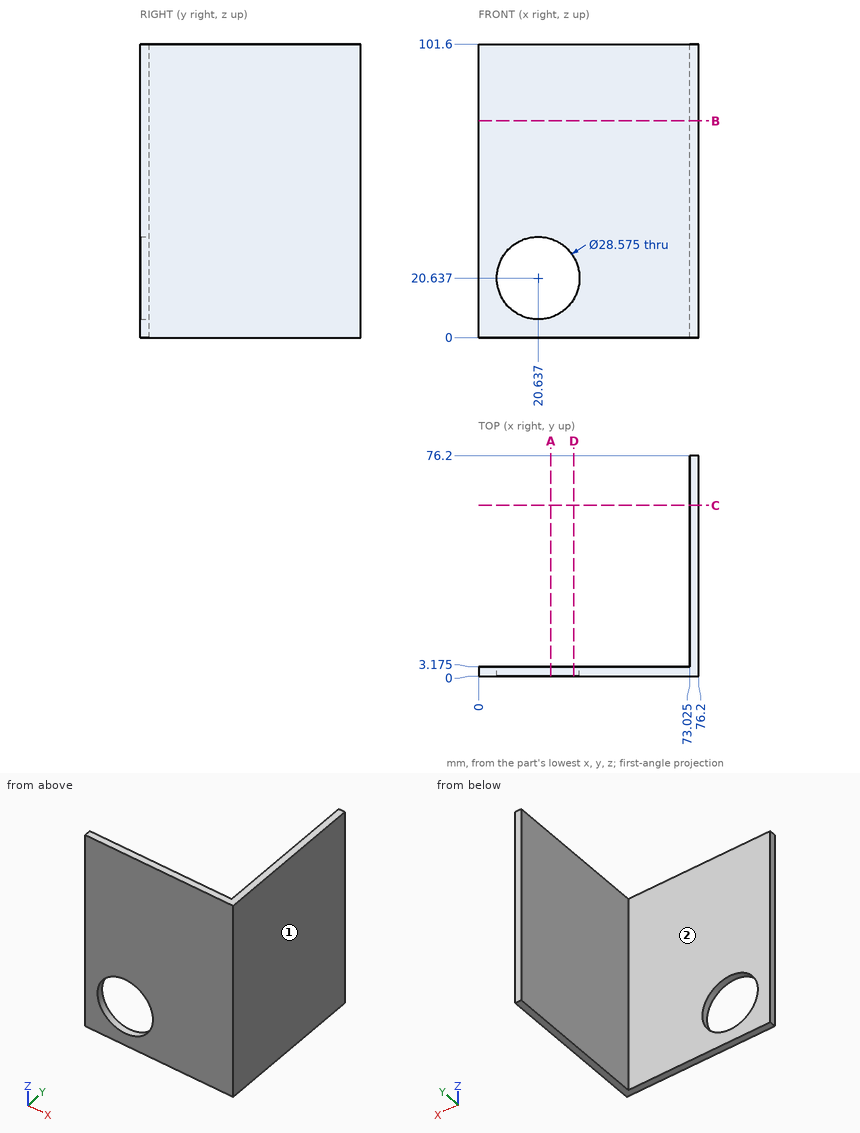
Could you check a few things on this drawing? It's one solid part, dimensions in mm from its lowest x, y, z. A direction names the side the tool comes from. Coordinates: 2 decimals unless noted, no trailing zeros. Write each loop counter-clockwise with the first axis right and the second up, starting at its lowest first coordinate (ties: lowest second). Pieces come first, ordered by that corner, then holes. Notation, with made-up numbers: M 52.5,77.25 L 87.5,77.25 A20 ccw 87.5,93.25 Z; hole C 2.25,53.5 d11. An arc over 180 degrees is marked long. Answer as CSV lines item,"result". Start each with the question number.
Q1. For the marked faces 1 and 2, which set-ups out of +Z, -Z, +X, -X, +Y, -Y let a thin tool reach every point of the face, with its end or its side?
Q2. Suppose I cut it at D-D, the plane x = 33. List the corners of the cut face in (y, z) for me (1 decimal).
Q3. Suppose I cut it at B-B, the plane z = 75. List the corners of the cut face in (x, y) for me (1 decimal).
Q4. Will these pins go through, and if not, where does the flat tip stop? pin 1 Ø5 at (x, z) = (18.5, 44) entering from +Y (1 decimal); pin 2 Ø8 at (x, z) = (47, 75) entering from -Y.
Q5. I need wall thicknesses on probe 1 along X at (y, z) = (22.5, 25) (1 decimal); probe 2 along Y at (x, z) = (47.5, 75.5) (1 decimal). Which ranges of each line are inside material? Lowest first, please. Write a range as [from, to].
Q6. Suppose I cut it at A-A, the plane x = 25. List the corners of the cut face in (y, z) for me (1 decimal).
Q7. Suppose I cut it at C-C, the plane y = 59. List the corners of the cut face in (x, z) for me (1 decimal).
Entries:
1,face 1,"+Z, -Z, +X, +Y, -Y"
1,face 2,"+Z, -Z, -X, +Y"
2,outline,"M 0,0 L 3.2,0 L 3.2,13.5 L 0,13.5 Z; M 0,27.8 L 3.2,27.8 L 3.2,101.6 L 0,101.6 Z"
3,outline,"M 0,0 L 76.2,0 L 76.2,76.2 L 73,76.2 L 73,3.2 L 0,3.2 Z"
4,pin 1,"stops at y = 3.2"
4,pin 2,"stops at y = 0"
5,probe 1,"x = [73, 76.2]"
5,probe 2,"y = [0, 3.2]"
6,outline,"M 0,0 L 3.2,0 L 3.2,7 L 0,7 Z; M 0,34.2 L 3.2,34.2 L 3.2,101.6 L 0,101.6 Z"
7,outline,"M 73,0 L 76.2,0 L 76.2,101.6 L 73,101.6 Z"
